Model file for the job. Use its own axes, mm. Give positions to 0.01 mm unless a question says otherwise; leave off trailing zeros. Order: outer loops, then holes, each group sorted by start corner. A loop starts at its lowest first (then second) coordinate and runs counter-clockwise, first axis right, second up. Notation, with made-up numbers: (-8.75, 4.5) - (2.25, 4.5) arc R18 ccw to (2.25, 38.5) - close; hole circle Ø9 at (84, -34.75). An arc over 180 degrees is marked (long way). Use CSV: the item, a comma, the result in double quotes. Start each with the question number.
(1) Band-saw the part on B-B, the plane y = 12.5. Count the separate pieces of the cut face and the enclosed holes in it, then the cut area to 3 significant figures.
(2) Probe L1, parallel to Y at x = 13, z = -10.25; L2, parallel to X at y = 9, z = -9; L3, parallel to X at y = 1, z = -4.5. List the from-to ranges inside material, lowest first.
(3) Drop a flat-ended pin along its axis: pin 1 Ø1.3 at (x, z) = (6, -9) entering from +Y. Give the stop position or say it passes through.
(4) Band-saw the part on A-A, the plane y = 7. Give the cut face in (x, z).
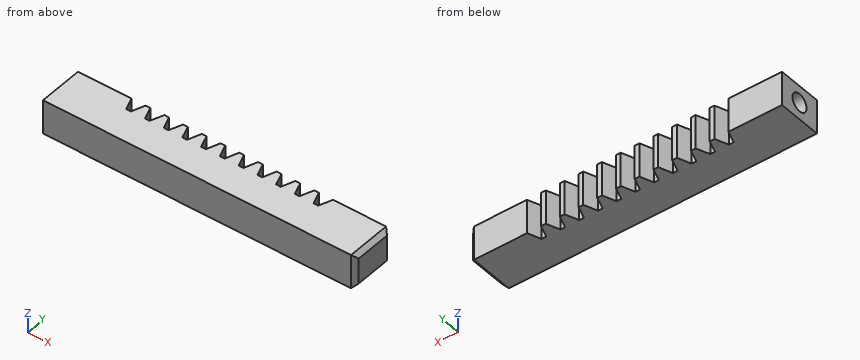
Autodesk Inventor part; units mm, degrees
ref_plane "YZ Plane" through (0, 0, 0) normal (1, 0, 0) x (0, 1, 0)
ref_plane "XZ Plane" through (0, 0, 0) normal (0, 1, 0) x (-1, 0, 0)
ref_plane "XY Plane" through (0, 0, 0) normal (0, 0, 1) x (1, 0, 0)
sketch "Sketch1" plane through (0, 0, 0) normal (0, 0, 1) x (1, 0, 0)
  line L0 (-77.7875, 0) -> (77.7875, 0)
  line L1 (0, -3.175) -> (0, 19.05)
  line L2 (-55.5625, 0) -> (55.5625, 0)
  line L3 (-55.5625, 0) -> (-55.5625, 15.875)
  line L4 (-55.5625, 15.875) -> (55.5625, 15.875)
  line L5 (55.5625, 15.875) -> (55.5625, 0)
  point P0 (0, 0)
  point P1 (0, 0)
  dimension "d0" = 111.125
  dimension "d1" = 15.875
extrude "Extrusion1" add sketch "Sketch1" against normal blind 12.1285
sketch "Sketch2" plane through (0, 0, 0) normal (0, 0, 1) x (1, 0, 0)
  line L0 (-55.5625, 15.875) -> (55.5625, 15.875)
  line L1 (-55.5625, 15.875) -> (-36.5125, 15.875)
  line L2 (-36.5125, 15.875) -> (-34.8577, 11.3284)
  line L3 (-34.8577, 11.3284) -> (-33.1851, 11.3284)
  line L4 (-33.1851, 11.3284) -> (-31.5303, 15.875)
  line L5 (-31.5303, 15.875) -> (-29.8577, 15.875)
  line L6 (55.5625, 15.875) -> (-55.5625, 15.875) construction
  line L7 (-55.5625, 15.875) -> (-55.5625, 0)
  line L8 (55.5625, 15.875) -> (36.5125, 15.875)
  line L9 (-29.845, 15.875) -> (-28.1902, 11.3284)
  line L10 (-28.1902, 11.3284) -> (-26.5176, 11.3284)
  line L11 (-26.5176, 11.3284) -> (-24.8628, 15.875)
  line L12 (-24.8628, 15.875) -> (-23.1902, 15.875)
  line L13 (-23.1775, 15.875) -> (-21.5227, 11.3284)
  line L14 (-21.5227, 11.3284) -> (-19.8501, 11.3284)
  line L15 (-19.8501, 11.3284) -> (-18.1953, 15.875)
  line L16 (-18.1953, 15.875) -> (-16.5227, 15.875)
  line L17 (-16.51, 15.875) -> (-14.8552, 11.3284)
  line L18 (-14.8552, 11.3284) -> (-13.1826, 11.3284)
  line L19 (-13.1826, 11.3284) -> (-11.5278, 15.875)
  line L20 (-11.5278, 15.875) -> (-9.8552, 15.875)
  line L21 (-9.8425, 15.875) -> (-8.1877, 11.3284)
  line L22 (-8.1877, 11.3284) -> (-6.5151, 11.3284)
  line L23 (-6.5151, 11.3284) -> (-4.8603, 15.875)
  line L24 (-4.8603, 15.875) -> (-3.1877, 15.875)
  line L25 (-3.175, 15.875) -> (-1.5202, 11.3284)
  line L26 (-1.5202, 11.3284) -> (0.1524, 11.3284)
  line L27 (0.1524, 11.3284) -> (1.8072, 15.875)
  line L28 (1.8072, 15.875) -> (3.4798, 15.875)
  line L29 (3.4925, 15.875) -> (5.1473, 11.3284)
  line L30 (5.1473, 11.3284) -> (6.8199, 11.3284)
  line L31 (6.8199, 11.3284) -> (8.4747, 15.875)
  line L32 (8.4747, 15.875) -> (10.1473, 15.875)
  line L33 (10.16, 15.875) -> (11.8148, 11.3284)
  line L34 (11.8148, 11.3284) -> (13.4874, 11.3284)
  line L35 (13.4874, 11.3284) -> (15.1422, 15.875)
  line L36 (15.1422, 15.875) -> (16.8148, 15.875)
  line L37 (16.8275, 15.875) -> (18.4823, 11.3284)
  line L38 (18.4823, 11.3284) -> (20.1549, 11.3284)
  line L39 (20.1549, 11.3284) -> (21.8097, 15.875)
  line L40 (21.8097, 15.875) -> (23.4823, 15.875)
  line L41 (23.495, 15.875) -> (25.1498, 11.3284)
  line L42 (25.1498, 11.3284) -> (26.8224, 11.3284)
  line L43 (26.8224, 11.3284) -> (28.4772, 15.875)
  line L44 (28.4772, 15.875) -> (30.1498, 15.875)
  line L45 (30.1625, 15.875) -> (31.8173, 11.3284)
  line L46 (31.8173, 11.3284) -> (33.4899, 11.3284)
  line L47 (33.4899, 11.3284) -> (35.1447, 15.875)
  line L48 (35.1447, 15.875) -> (36.8173, 15.875)
  point P0 (0, 0)
  point P1 (-35.6851, 13.6017)
  point P2 (-32.3577, 13.6017)
  point P3 (-29.0176, 13.6017)
  point P4 (-25.6902, 13.6017)
  point P5 (-22.3501, 13.6017)
  point P6 (-19.0227, 13.6017)
  point P7 (-15.6826, 13.6017)
  point P8 (-12.3552, 13.6017)
  point P9 (-9.0151, 13.6017)
  point P10 (-5.6877, 13.6017)
  point P11 (-2.3476, 13.6017)
  point P12 (0.9798, 13.6017)
  point P13 (4.3199, 13.6017)
  point P14 (7.6473, 13.6017)
  point P15 (10.9874, 13.6017)
  point P16 (14.3148, 13.6017)
  point P17 (17.6549, 13.6017)
  point P18 (20.9823, 13.6017)
  point P19 (24.3224, 13.6017)
  point P20 (27.6498, 13.6017)
  point P21 (30.9899, 13.6017)
  point P22 (34.3173, 13.6017)
  dimension "d4" = 19.05
  dimension "d5" = 6.6548
  dimension "d6" = 20
  dimension "d7" = 4.5466
  dimension "d12" = 6.6675
extrude "Extrusion2" cut sketch "Sketch2" against normal through all
sketch "Sketch3" plane through (-55.5625, 0, 0) normal (-1, 0, 0) x (0, 0, 1)
  circle A0 centre (-6.0642, 7.9375) radius 3.175
  line L0 (-12.1285, 0) -> (-12.1285, 15.875)
  line L1 (0, 15.875) -> (-12.1285, 15.875)
  point P0 (0, 0)
  point P1 (-12.1285, 7.9375)
  point P2 (-6.0642, 15.875)
  dimension "d19" = 6.35
extrude "Extrusion3" cut sketch "Sketch3" against normal blind 15.875
chamfer "Chamfer1" distance 1.524 angle 45 4 edges at (55.5625, 15.875, -6.0642) (55.5625, 7.9375, 0) (55.5625, 0, -6.0642) (55.5625, 7.9375, -12.1285)
properties part number "Ch7(5) Part 11 Rack"
Answer block:
1,separate pieces,"12"
1,enclosed holes,"0"
1,area,"1,010 mm2"
2,L1,"y = 0 to 11.33"
2,L2,"x = -39.69 to 55.56"
2,L3,"x = -55.56 to 55.04"
3,pin 1,"stops at y = 11.33"
4,outline,"(-55.56, -12.13) - (54.04, -12.13) - (55.56, -10.6) - (55.56, -1.52) - (54.04, 0) - (-55.56, 0) - (-55.56, -3.03) - (-39.69, -3.03) - (-39.69, -9.1) - (-55.56, -9.1) - close"
